Can you work these out from the model? Positions are in its coordinate system, mm. Round coordinates to 2 decimals unless told otherwise and drop trailing zeros. Write each loop counter-clockwise with the first axis right and the second up, starting at its lowest first coordinate (ties: lowest second). Pieces come first, ordered by that corner, then holes. Notation, with made-up numbers: (54, 20.5) -> (71, 20.5) arc R8 cw to (71, 32.5) -> close; hole circle Ø7 at (77.5, 63.5). An arc over 180 degrees is marked (long way). Use CSV: the item, a comma, the result in double quotes.
```python
from build123d import *

# Parameters (mm, degrees)
CYLINDER006_R     = 4.7
CYLINDER006_DEPTH = 6
CYLINDER003_R     = 1.4
CYLINDER003_DEPTH = 10
CYLINDER004_R     = 1.4
CYLINDER004_DEPTH = 10
CYLINDER005_R     = 1.4
CYLINDER005_DEPTH = 10
CYLINDER002_R     = 1.4
CYLINDER002_DEPTH = 10
CYLINDER_R        = 12
CYLINDER_DEPTH    = 4


with BuildPart() as cylinder006:
    # Cylinder006 → Cylinder006 (new body)
    with BuildSketch(Plane.XY.offset(-1)):
        Circle(CYLINDER006_R)
    extrude(amount=CYLINDER006_DEPTH)


with BuildPart() as cylinder003:
    # Cylinder003 → Cylinder003 (new body)
    with BuildSketch(Plane(origin=(8.5, 0, -1), x_dir=(1, 0, 0), z_dir=(0, 0, 1))):
        Circle(CYLINDER003_R)
    extrude(amount=CYLINDER003_DEPTH)


with BuildPart() as cylinder004:
    # Cylinder004 → Cylinder004 (new body)
    with BuildSketch(Plane(origin=(0, 8.5, -1), x_dir=(1, 0, 0), z_dir=(0, 0, 1))):
        Circle(CYLINDER004_R)
    extrude(amount=CYLINDER004_DEPTH)


with BuildPart() as cylinder005:
    # Cylinder005 → Cylinder005 (new body)
    with BuildSketch(Plane(origin=(0, -8.5, -1), x_dir=(1, 0, 0), z_dir=(0, 0, 1))):
        Circle(CYLINDER005_R)
    extrude(amount=CYLINDER005_DEPTH)


with BuildPart() as cylinder002:
    # Cylinder002 → Cylinder002 (new body)
    with BuildSketch(Plane(origin=(-8.5, 0, -1), x_dir=(1, 0, 0), z_dir=(0, 0, 1))):
        Circle(CYLINDER002_R)
    extrude(amount=CYLINDER002_DEPTH)


with BuildPart() as obj1:
    # Cylinder → Cylinder (new body)
    with BuildSketch(Plane.XY):
        Circle(CYLINDER_R)
    extrude(amount=CYLINDER_DEPTH)

    # Cut: cut Cylinder002
    add(cylinder002.part, mode=Mode.SUBTRACT)

    # Cut001: cut Cylinder005
    add(cylinder005.part, mode=Mode.SUBTRACT)

    # Cut002: cut Cylinder004
    add(cylinder004.part, mode=Mode.SUBTRACT)

    # Cut003: cut Cylinder003
    add(cylinder003.part, mode=Mode.SUBTRACT)

    # Cut004: cut Cylinder006
    add(cylinder006.part, mode=Mode.SUBTRACT)


solid = obj1.part
```
Q1. Suppose I cut it at C-C (y = -7.5). Write out the boundary of the cut face in (x, z).
Resolved:
outline,"(-9.37, 0) -> (-0.98, 0) -> (-0.98, 4) -> (-9.37, 4) -> close; (0.98, 0) -> (9.37, 0) -> (9.37, 4) -> (0.98, 4) -> close"
Q2. Will these pins go through, and if not, where does the flat tip stop? P1, Ø2, axis at x = -8.5, y = 0, coming from the -Z side; P2, Ø2, axis at x = 8.5, z = 2, coming from the -Y side; P3, Ø1, axis at x = -1, z = 0.5, coming from the -Y side; P4, Ø1, axis at y = 1.5, z = 2.5, coming from the +X side.
Resolved:
P1,"passes through"
P2,"stops at y = -9.37"
P3,"stops at y = -11.99"
P4,"stops at x = 11.96"
Q3. If we mould it in two halves opening along X, with no side actions, what happens to faces 1 (the face through (5, 0, 0)), 2 (the face through (-11.99, 0.53, 1.97)), 3 (the face through (-0.303, -9.867, 1.972))? For each: released by +X, released by -X, zero draft, split by the parting line, or undercut.
Resolved:
face 1,"zero draft"
face 2,"split by the parting line"
face 3,"undercut"
Q4. Suppose I cut it at A-A (y = 0). Write out the boundary of the cut face in (x, z).
Resolved:
outline,"(-12, 0) -> (-9.9, 0) -> (-9.9, 4) -> (-12, 4) -> close; (-7.1, 0) -> (-4.7, 0) -> (-4.7, 4) -> (-7.1, 4) -> close; (4.7, 0) -> (7.1, 0) -> (7.1, 4) -> (4.7, 4) -> close; (9.9, 0) -> (12, 0) -> (12, 4) -> (9.9, 4) -> close"
Q5. Suppose I cut it at B-B (x = -0.5). Write out the boundary of the cut face in (y, z).
Resolved:
outline,"(-11.99, 0) -> (-9.81, 0) -> (-9.81, 4) -> (-11.99, 4) -> close; (-7.19, 0) -> (-4.67, 0) -> (-4.67, 4) -> (-7.19, 4) -> close; (4.67, 0) -> (7.19, 0) -> (7.19, 4) -> (4.67, 4) -> close; (9.81, 0) -> (11.99, 0) -> (11.99, 4) -> (9.81, 4) -> close"
Q6. Please list where these lines run through material, in increasing order: probe 1 along Y at (x, z) = (-0.75, 3.65); probe 2 along Y at (x, z) = (9.5, 1.95); probe 3 along X at (y, z) = (-4, 3.3).
Resolved:
probe 1,"y = -11.98 to -9.68, -7.32 to -4.64, 4.64 to 7.32, 9.68 to 11.98"
probe 2,"y = -7.33 to -0.98, 0.98 to 7.33"
probe 3,"x = -11.31 to -2.47, 2.47 to 11.31"
Q7. Suppose I cut it at D-D (z = 1.85). Write out the boundary of the cut face in (x, y).
Resolved:
outline,"circle Ø24 at (0, 0); hole circle Ø2.8 at (-8.5, 0); hole circle Ø9.4 at (0, 0); hole circle Ø2.8 at (0, -8.5); hole circle Ø2.8 at (0, 8.5); hole circle Ø2.8 at (8.5, 0)"
